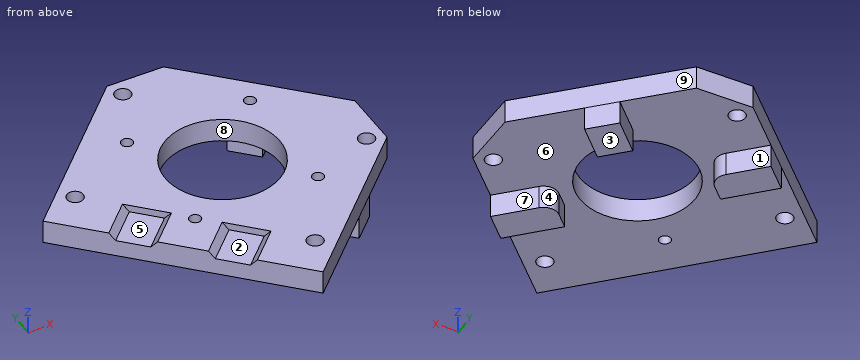
Solid Edge part; units mm, degrees
sketch "Sketch1" plane through (0, 0, 24) normal (0, 0, 1) x (1, 0, 0)
  circle A0 centre (-13, 13) radius 1.2295
  circle A1 centre (13, 13) radius 1.2295
  circle A2 centre (13, -13) radius 1.2295
  circle A3 centre (-13, -13) radius 1.2295
  circle A4 centre (0, 0) radius 12
  circle A5 centre (-6.6628, 26.0299) radius 1.7
  circle A6 centre (26.3661, -7.408) radius 1.7
  circle A7 centre (-29.2628, 3.4479) radius 1.7
  circle A8 centre (3.2628, -29.4479) radius 1.7
  line L0 (0, -38.3993) -> (29.8661, -8.8693)
  line L1 (29.8661, -8.8693) -> (29.9361, 3.4929)
  line L2 (3.899, 29.5299) -> (29.9361, 3.4929)
  line L3 (3.899, 29.5299) -> (-8.101, 29.5299)
  line L4 (-8.101, 29.5299) -> (-37.9671, 0)
  line L5 (-37.9671, 0) -> (0, -38.3993)
  dimension "D1" = 37.9671
  dimension "D2" = 8.101
  dimension "D3" = 6.6628
extrude "ExtrudedProtrusion_2" add sketch "Sketch1" against normal blind 5
sketch "Sketch2" plane through (-3.908, -4.4218, 19) normal (0, 0, -1) x (-0.7111, -0.7031, 0)
  line L0 (-2.3838, 27.091) -> (-9.1838, 27.091)
  line L1 (-9.1838, 27.091) -> (-9.1838, 18.3811)
  arc A0 (-6.1838, 15.3811) -> (-9.1838, 18.3811) centre (-6.1838, 18.3811) cw
  line L2 (-6.1838, 15.3811) -> (-2.3838, 15.3811)
  line L3 (-2.3838, 15.3811) -> (-2.3838, 27.091)
  line L4 (-2.5919, -26.909) -> (-9.3919, -26.909)
  line L5 (-9.3919, -26.909) -> (-9.3919, -17.5879)
  arc A1 (-9.3919, -17.5879) -> (-6.3919, -14.5879) centre (-6.3919, -17.5879) cw
  line L6 (-6.3919, -14.5879) -> (-2.5919, -14.5879)
  line L7 (-2.5919, -14.5879) -> (-2.5919, -26.909)
  line L8 (-29.5446, -2.8696) -> (-29.5061, 3.9303)
  line L9 (-29.5061, 3.9303) -> (-20.8532, 3.8814)
  line L10 (-20.8532, 3.8814) -> (-20.8917, -2.9185)
  line L11 (-20.8917, -2.9185) -> (-29.5446, -2.8696)
extrude "ExtrudedProtrusion_4" add sketch "Sketch2" along normal blind 5
sketch "Sketch3" plane through (-18.9835, -19.1996, 21.5) normal (-0.7111, -0.7031, 0) x (-0.7031, 0.7111, 0)
  line L0 (-14.3229, -2.5) -> (-13, -1)
  line L1 (-13, -1) -> (-6.2152, -1)
  line L2 (-6.2152, -1) -> (-4.8924, -2.5)
  line L3 (-4.8924, -2.5) -> (-14.3229, -2.5)
  line L4 (14.3229, -2.5) -> (4.8924, -2.5)
  line L5 (4.8924, -2.5) -> (6.2152, -1)
  line L6 (6.2152, -1) -> (13, -1)
  line L7 (13, -1) -> (14.3229, -2.5)
  dimension "D1" = 14.3229
  dimension "D2" = 6.2152
extrude "Cutout1" cut sketch "Sketch3" against normal blind 9
properties material "ABS Plastic, high impact"
For this review, take the finished solid that the model builds, in its own axes (mm). Face numbers are marked on the shaded views. A direction names the side the tool comes from. Round coordinates to 2 decimals unless told otherwise and drop trailing zeros. Order: outer loops, then holes, each group sorted by start corner. A loop starts at its lowest first (then second) coordinate and runs counter-clockwise, first axis right, second up. Notation, with made-up numbers: M 79,-24 L 108,-24 A23 cw 108,-10 Z; hole C 78,-34.75 d4. An arc over 180 degrees is marked long. Use a Markdown table: item, result. Add a question column.
Item 1: Mouldability with a two-part tool opening along X and no side actions: class the marked faces 1, 2, 3 and 4 as released by +X, released by -X, zero draft, split by the parting line, or undercut.
Item 2: Add section B-B, the plane y = -25.5. Give the boundary of the cut face in (x, z).
Item 3: To check wall thickness, follow line 1 along Y through (x, z) = (13.5, 22.75); line 2 along Y through (x, z) = (-13, 21.6); line 3 along Z through (x, y) = (18, 4). State the ranges of each line that lie inside material, in increasing order.
Item 4: Insertion check: pin 1 (4 mm diameter, centred on x = -13, y = -13, fed in from -Z); pin 2 (0.7 mm diameter, centred on x = -12.5, y = 13, fed in from +Z); pin 3 (2 mm diameter, centred on x = -26, z = 22, fed in from -Y). Each pin has a flat end and moves straight along its axis. Give the tip position at first contact, or say it passes through.
Item 5: Add section A-A, the plane z = 17.5. Give the boundary of the cut face in (x, y) (3 decimals).
Item 6: Tool access review of the marked faces 5, 6, 7, 8 and 9: name each direction out of +Z, -Z, +X, -X, +Y, -Y from which nothing blocks a thin tool from reaching the whole face with its end or side.
Geometry results:
| question | item | result |
|---|---|---|
| 1 | face 1 | undercut |
| 1 | face 2 | undercut |
| 1 | face 3 | zero draft |
| 1 | face 4 | split by the parting line |
| 2 | outline | M -12.75,19 L 13.05,19 L 13.05,24 L -4.98,24 L -6.87,22.5 L -12.75,22.5 Z |
| 3 | line 1 | y = -25.05 to -14.12, -11.88 to 11.88, 14.12 to 19.93 |
| 3 | line 2 | y = -25.25 to -14.23, -11.77 to 11.77, 14.23 to 24.69 |
| 3 | line 3 | z = 19 to 24 |
| 4 | pin 1 | stops at z = 19 |
| 4 | pin 2 | stops at z = 19 |
| 4 | pin 3 | stops at y = -13.11 |
| 5 | outline | M -21.26,16.519 L -13.027,8.192 L -10.325,10.863 A3 ccw -10.301,15.106 L -16.425,21.3 Z; M 8.192,-12.973 L 16.855,-21.734 L 21.69,-16.953 L 15.137,-10.325 A3 ccw 10.894,-10.301 Z; M 8.192,13 L 13,8.192 L 19.119,14.31 L 14.31,19.119 Z |
| 6 | face 5 | +Z |
| 6 | face 6 | -Z |
| 6 | face 7 | -Z, +X |
| 6 | face 8 | +Z, -Z |
| 6 | face 9 | +Z, -Z, +X, +Y |
